Work out the finished part from the listing and answer in its coordinate system (mm). Face numbers are marked on the shaded views. A direction names the side the tool comes from. Coordinates: 2 decimals unless noted, no trailing zeros. Loops run counter-clockwise (first coordinate to the right, second up) from the corner with the lowest first, then second, coordinate; pieces in that order, holes last. Notation, with made-up numbers: (39, 28.25) - (49, 28.25) arc R20 cw to (49, 40.25) - close; hole circle Ø7 at (-35, -27.5). An arc over 180 degrees is marked (long way). Write each question's results on one line, items separated by ' | '. Start each with the question number.
Item 1: Each of these flat-tipped pins is pushed along its axis until it touches: pin 1 Ø10 at (x, y) = (9, 0) entering from +Z; pin 2 Ø0.5 at (x, z) = (13.5, 2.5) entering from -Y; pin 3 Ø2 at (x, z) = (35, 2) entering from +Y; pin 4 Ø4 at (x, y) = (30, 6.5) entering from +Z. Where does it stop, or does it pass through?
Item 2: Consider probe 1 along Y at (x, z) = (34, 2.75); probe 2 along X at (y, z) = (6, 1.5); probe 3 along Z at (x, y) = (8, -5). Determine where each line is inside the solid, lowest interval first. Write a range as [from, to].
Item 3: A tool of negligible diameter and unlimited length cuts with its end or side. For the marked faces 1, 2, 3, 4 and 5, from which of +Z, -Z, +X, -X, +Y, -Y can it reach the whole face along a straight path? Write none if from no direction.
Item 4: Section A-A, the plane x = 30 is taken. Write down the section's boundary in (y, z).
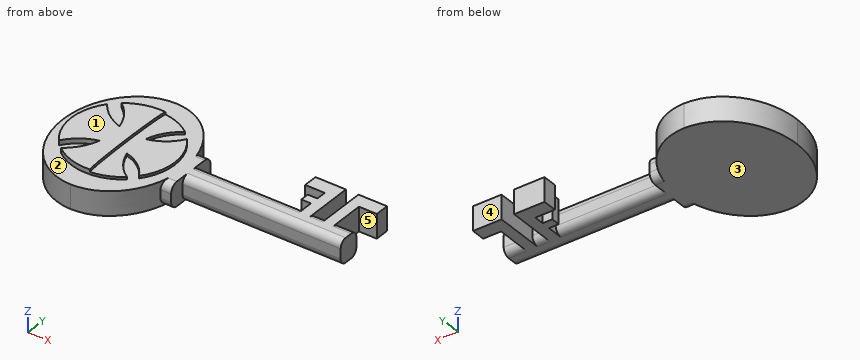
from build123d import *

# Parameters (mm, degrees)
PAD002_DEPTH = 35
PAD003_DEPTH = 4
PAD004_DEPTH = 5
PAD005_DEPTH = 5
PAD_DEPTH    = 1
POCKET_DEPTH = 0.5


with BuildPart() as part:
    # Sketch002 → Pad002 (new body)
    with BuildSketch(Plane.YZ.offset(46.87)):
        with BuildLine():
            Line((-0.77, 5), (0.77, 5))
            ThreePointArc((2.22, 3.55), (1.795305, 4.575305), (0.77, 5))
            Line((2.22, 3.55), (2.22, 1.45))
            ThreePointArc((0.77, 0), (1.795305, 0.424695), (2.22, 1.45))
            Line((0.77, 0), (-0.77, 0))
            ThreePointArc((-2.22, 1.45), (-1.795305, 0.424695), (-0.77, 0))
            Line((-2.22, 1.45), (-2.22, 3.55))
            ThreePointArc((-0.77, 5), (-1.795305, 4.575305), (-2.22, 3.55))
        make_face()
    extrude(amount=-PAD002_DEPTH)

    # Sketch003 → Pad003 (join)
    with BuildSketch(Plane.YZ.offset(14)):
        with BuildLine():
            Line((-3.803555, 0), (4.066445, 0))
            ThreePointArc((4.066445, 0), (5.233171, 0.483274), (5.716445, 1.65))
            Line((5.716445, 1.65), (5.716445, 3.35))
            ThreePointArc((5.716445, 3.35), (5.233171, 4.516726), (4.066445, 5))
            Line((4.066445, 5), (-3.803555, 5))
            ThreePointArc((-3.803555, 5), (-4.970281, 4.516726), (-5.453555, 3.35))
            Line((-5.453555, 3.35), (-5.453555, 1.65))
            ThreePointArc((-5.453555, 1.65), (-4.970281, 0.483274), (-3.803555, 0))
        make_face()
    extrude(amount=-PAD003_DEPTH)

    # Sketch005 → Pad004 (join)
    with BuildSketch(Plane.XY):
        with BuildLine():
            add(Edge.make_bspline(
                [(-0.016421, 15.055976), (-1.51312, 15.047784), (-3.00857, 14.811385), (-4.467156, 14.346958), (-5.853346, 13.665527), (-7.137203, 12.788252), (-8.299907, 11.744186), (-9.335169, 10.555337), (-10.232104, 9.242889), (-10.987087, 7.827952), (-11.593837, 6.330415), (-12.049258, 4.771197), (-12.350633, 3.170976), (-12.496836, 1.550706), (-12.487972, -0.068717)],
                knots=[0, 0, 0, 0, 0, 0, 0, 0, 0, 0, 0, 0, 0, 0, 0, 1.570796, 1.570796, 1.570796, 1.570796, 1.570796, 1.570796, 1.570796, 1.570796, 1.570796, 1.570796, 1.570796, 1.570796, 1.570796, 1.570796, 1.570796], degree=14))
            add(Edge.make_bspline(
                [(-12.487972, -0.068717), (-12.479108, -1.688139), (-12.315176, -3.306712), (-11.996302, -4.903537), (-11.523839, -6.457677), (-10.900731, -7.948482), (-10.130305, -9.35507), (-9.219056, -10.65762), (-8.170841, -11.835064), (-6.996777, -12.86634), (-5.703394, -13.729507), (-4.309827, -14.395723), (-2.846245, -14.844155), (-1.348296, -15.064169), (0.148403, -15.055976)],
                knots=[1.570796, 1.570796, 1.570796, 1.570796, 1.570796, 1.570796, 1.570796, 1.570796, 1.570796, 1.570796, 1.570796, 1.570796, 1.570796, 1.570796, 1.570796, 3.141593, 3.141593, 3.141593, 3.141593, 3.141593, 3.141593, 3.141593, 3.141593, 3.141593, 3.141593, 3.141593, 3.141593, 3.141593, 3.141593, 3.141593], degree=14))
            add(Edge.make_bspline(
                [(0.148403, -15.055976), (1.645102, -15.047784), (3.140552, -14.811385), (4.599138, -14.346958), (5.985328, -13.665527), (7.269185, -12.788252), (8.431889, -11.744186), (9.467151, -10.555337), (10.364086, -9.242889), (11.119069, -7.827952), (11.725819, -6.330415), (12.18124, -4.771197), (12.482615, -3.170976), (12.628818, -1.550706), (12.619954, 0.068717)],
                knots=[3.141593, 3.141593, 3.141593, 3.141593, 3.141593, 3.141593, 3.141593, 3.141593, 3.141593, 3.141593, 3.141593, 3.141593, 3.141593, 3.141593, 3.141593, 4.712389, 4.712389, 4.712389, 4.712389, 4.712389, 4.712389, 4.712389, 4.712389, 4.712389, 4.712389, 4.712389, 4.712389, 4.712389, 4.712389, 4.712389], degree=14))
            add(Edge.make_bspline(
                [(12.619954, 0.068717), (12.61109, 1.688139), (12.447158, 3.306712), (12.128284, 4.903537), (11.655821, 6.457677), (11.032713, 7.948482), (10.262287, 9.35507), (9.351038, 10.65762), (8.302823, 11.835064), (7.128759, 12.86634), (5.835376, 13.729507), (4.441809, 14.395723), (2.978227, 14.844155), (1.480278, 15.064169), (-0.016421, 15.055976)],
                knots=[4.712389, 4.712389, 4.712389, 4.712389, 4.712389, 4.712389, 4.712389, 4.712389, 4.712389, 4.712389, 4.712389, 4.712389, 4.712389, 4.712389, 4.712389, 6.283185, 6.283185, 6.283185, 6.283185, 6.283185, 6.283185, 6.283185, 6.283185, 6.283185, 6.283185, 6.283185, 6.283185, 6.283185, 6.283185, 6.283185], degree=14))
        make_face()
    extrude(amount=PAD004_DEPTH)

    # Sketch006 → Pad005 (join)
    with BuildSketch(Plane.XY):
        Polygon((43.121773, 8.076345), (43.121773, 0.549987), (40.917084, 0.549987), (40.917084, 10.96525), (46.846939, 10.96525), (46.846939, 8.076345), align=None)
        Polygon((31.984285, 10.96525), (38.294262, 10.96525), (38.294262, 0.626011), (36.051559, 0.626011), (36.051559, 4.123106), (34.036926, 4.123106), (34.036926, 5.947678), (36.051559, 5.947678), (36.051559, 8.038333), (31.984285, 8.038333), align=None)
    extrude(amount=PAD005_DEPTH)

    # Sketch (on Face46 of Pad005) → Pad (join)
    with BuildSketch(Plane(origin=(0, 0, 5), x_dir=(0, -1, 0), z_dir=(0, 0, 1))):
        with BuildLine():
            ThreePointArc((-8.409153, 6.728971), (-10.769324, 0.120636), (-8.557777, -6.53891))
            ThreePointArc((-2.682549, -2.707352), (-5.947717, -4.120868), (-8.557777, -6.53891))
            ThreePointArc((-6.84041, -8.318755), (-4.297701, -5.856698), (-2.682549, -2.707352))
            ThreePointArc((-6.84041, -8.318755), (-0.069564, -10.769775), (6.732378, -8.406425))
            ThreePointArc((2.777161, -2.829888), (4.233029, -5.988206), (6.732378, -8.406425))
            ThreePointArc((8.371362, -6.775928), (5.903039, -4.336809), (2.777161, -2.829888))
            ThreePointArc((8.371362, -6.775928), (10.769725, 0.076933), (8.273705, 6.894832))
            ThreePointArc((2.555971, 2.675341), (5.803156, 4.258886), (8.273705, 6.894832))
            ThreePointArc((6.851023, 8.310017), (4.104112, 5.949562), (2.555971, 2.675341))
            ThreePointArc((6.851023, 8.310017), (-0.022073, 10.769977), (-6.885028, 8.281865))
            ThreePointArc((-2.780082, 2.669729), (-4.25796, 5.896079), (-6.885028, 8.281865))
            ThreePointArc((-8.409153, 6.728971), (-5.958868, 4.194233), (-2.780082, 2.669729))
        make_face()
    extrude(amount=PAD_DEPTH)

    # Sketch009 (on Face74 of Pad) → Pocket (cut)
    with BuildSketch(Plane(origin=(1, 0, 6), x_dir=(0, -1, 0), z_dir=(0, 0, 1))):
        with BuildLine():
            add(Edge.make_bspline(
                [(-10.77411, 0), (-10.77411, -0.438108), (0, -0.438108), (10.77411, -0.438108), (10.77411, 0)],
                knots=[0, 0, 0, 1.570796, 1.570796, 3.141593, 3.141593, 3.141593], degree=2, weights=[1, 0.707107, 1, 0.707107, 1]))
            Line((10.77411, 0), (10.77411, 9.970053))
            Line((10.77411, 9.970053), (-10.77411, 9.970053))
            Line((-10.77411, 9.970053), (-10.77411, 0))
        make_face()
    extrude(amount=-POCKET_DEPTH, mode=Mode.SUBTRACT)


solid = part.part
Answer key:
1) pin 1: stops at z = 5.5 | pin 2: stops at y = -5.45 | pin 3: stops at y = 10.97 | pin 4: passes through
2) probe 1: y = [-2.22, 2.22], [8.04, 10.97] | probe 2: x = [-11.47, 11.58], [36.05, 38.29], [40.92, 43.12] | probe 3: z = [0, 5.5]
3) face 1: +Z, +X, -X, +Y, -Y | face 2: +Z | face 3: -Z, +X, -X, +Y, -Y | face 4: +Z, -Z, +X, +Y | face 5: +Z, -Z, +X
4) outline: (-2.22, 1.45) arc R1.45 ccw to (-0.77, 0) - (0.77, 0) arc R1.45 ccw to (2.22, 1.45) - (2.22, 3.55) arc R1.45 ccw to (0.77, 5) - (-0.77, 5) arc R1.45 ccw to (-2.22, 3.55) - close
